```python
from build123d import *

# Parameters (mm, degrees)
SKETCH1_W           = 21.844
SKETCH1_H           = 127
SKETCH1_R           = 3.175
BOSS_EXTRUDE1_DEPTH = 23.749
SKETCH3_W           = 5.531865031
SKETCH3_H           = 127
CUT_EXTRUDE2_DEPTH  = 4.7625


with BuildPart() as part:
    # Sketch1 → Boss-Extrude1 (new body)
    with BuildSketch(Plane(origin=(0, 0, 0), x_dir=(1, 0, 0), z_dir=(0, 1, 0))):
        Rectangle(SKETCH1_W, SKETCH1_H)
        with Locations(Location((0, 31.75, 0), (0, 0, 90))):
            Circle(SKETCH1_R, mode=Mode.SUBTRACT)
        with Locations(Location((0, 47.625, 0), (0, 0, 90))):
            Circle(SKETCH1_R, mode=Mode.SUBTRACT)
        with Locations(Location((0, -31.75, 0), (0, 0, 90))):
            Circle(SKETCH1_R, mode=Mode.SUBTRACT)
        with Locations(Location((0, -47.625, 0), (0, 0, 90))):
            Circle(SKETCH1_R, mode=Mode.SUBTRACT)
    extrude(amount=BOSS_EXTRUDE1_DEPTH)

    # Sketch3 → Cut-Extrude2 (cut)
    with BuildSketch(Plane(origin=(0, 23.749, 0), x_dir=(1, 0, 0), z_dir=(0, 1, 0))):
        with Locations((-8.156067484, 0)):
            Rectangle(SKETCH3_W, SKETCH3_H)
        with Locations((8.156067484, 0)):
            Rectangle(SKETCH3_W, SKETCH3_H)
    extrude(amount=-CUT_EXTRUDE2_DEPTH, mode=Mode.SUBTRACT)


solid = part.part
```
Verification items for the finished model (mm, model axes). A direction names the side the tool comes from. Give positions to 0.01 mm unless a question says otherwise; leave off trailing zeros. Write each loop counter-clockwise with the first axis right and the second up, starting at its lowest first coordinate (ties: lowest second). Pieces come first, ordered by that corner, then holes. Notation, with made-up numbers: (50.5, 25) - (105.5, 25) arc R18 ccw to (105.5, 58) - close; hole circle Ø5 at (18, 51). An arc over 180 degrees is marked (long way). Put each result on its own line as item: value.
Q1. Scan lines: probe 1 along X at (y, z) = (16, 31.75) (3 decimals); probe 2 along Y at (x, z) = (7.75, -33.5); probe 3 along X at (y, z) = (14.25, 33). Record each from-to range of solid material in increasing order. Write a range as from..to.
Result:
probe 1: -10.922..-3.175, 3.175..10.922
probe 2: 0..18.99
probe 3: -10.92..-2.92, 2.92..10.92
Q2. Section check B-B on y = 22. Record the cut outline in (x, z) (3 decimals), and give its area (3 significant figures).
Result:
outline: (-5.39, -63.5) - (5.39, -63.5) - (5.39, 63.5) - (-5.39, 63.5) - close; hole circle Ø6.35 at (0, -47.625); hole circle Ø6.35 at (0, -31.75); hole circle Ø6.35 at (0, 31.75); hole circle Ø6.35 at (0, 47.625)
area: 1,240 mm2
Q3. Mould release check, pull along Z, two halves, no side actions. Record for faces 4 (the face through (-5.39, 21, 1)), 5 (the face through (0, 12, 63.5)), 6 (the face through (-0.954, 11.708, -50.653)): released by +Z, released by -Z, zero draft, split by the parting line, or undercut.
Result:
face 4: zero draft
face 5: released by +Z
face 6: undercut
Q4. Depth check by flat-ended pin: P1, Ø5, axis at x = 0, z = 31.75, coming from the +Y side (1 decimal); P2, Ø4, axis at y = 22.5, z = -24.5, coming from the +X side; P3, Ø3, axis at x = 8, z = 0, coming from the +Y side; P4, Ø1.4, axis at y = 21, z = 15.5, coming from the -X side. Enter the tip coordinate at first touch or a pass-through.
Result:
P1: through
P2: x = 5.39
P3: y = 18.99
P4: x = -5.39
Q5. Section check A-A on x = 0. Record the cut outline in (y, z) (3 decimals).
Result:
outline: (0, -63.5) - (23.749, -63.5) - (23.749, -50.8) - (0, -50.8) - close; (0, -44.45) - (23.749, -44.45) - (23.749, -34.925) - (0, -34.925) - close; (0, -28.575) - (23.749, -28.575) - (23.749, 28.575) - (0, 28.575) - close; (0, 34.925) - (23.749, 34.925) - (23.749, 44.45) - (0, 44.45) - close; (0, 50.8) - (23.749, 50.8) - (23.749, 63.5) - (0, 63.5) - close
Q6. Set-up check for faces 1 (the face through (-0.14, 11.71, 34.92)), 2 (the face through (8, 18.986, -1)), 3 (the face through (-8, 18.986, -1)): record each of +Z, -Z, +X, -X, +Y, -Y from which the full face is reachable in a straight line by a thin tool's end or side.
Result:
face 1: +Y, -Y
face 2: +Z, -Z, +X, +Y
face 3: +Z, -Z, -X, +Y
Q7. Section check C-C on z = -31.75. Record the cut outline in (x, y) (1 decimal), and give its area (3 significant figures).
Result:
outline: (-10.9, 0) - (-3.2, 0) - (-3.2, 23.7) - (-5.4, 23.7) - (-5.4, 19) - (-10.9, 19) - close; (3.2, 0) - (10.9, 0) - (10.9, 19) - (5.4, 19) - (5.4, 23.7) - (3.2, 23.7) - close
area: 315 mm2
Q8. Section check D-D on y = 14.25. Record the cut outline in (x, z) (3 decimals).
Result:
outline: (-10.922, -63.5) - (10.922, -63.5) - (10.922, 63.5) - (-10.922, 63.5) - close; hole circle Ø6.35 at (0, -47.625); hole circle Ø6.35 at (0, -31.75); hole circle Ø6.35 at (0, 31.75); hole circle Ø6.35 at (0, 47.625)
